Design review of the part built by this model. Coordinates are the model's own, in mm. A direction names the side the tool comes from. Coordinates: 2 decimals unless noted, no trailing zeros. Order: outer loops, then holes, each group sorted by start corner. A loop starts at its lowest first (then second) coordinate and runs counter-clockwise, first axis right, second up. Notation, with made-up numbers: M -5.5,8.5 L 31.5,8.5 A23 ccw 31.5,44.5 Z; hole C 83.25,-5 d3. An arc over 180 degrees is marked long. Use CSV: the item, a comma, the result in double quotes.
```python
from build123d import *

# Parameters (mm, degrees)
F1_DEPTH = 12.7
F2_W     = 101.6
F2_H     = 12.7
F3_DEPTH = 6.35
F4_R     = 5.08
F6_D     = 9.525
F8_D     = 6.35
F8_DEPTH = 5.08
F8_START = 0.3707141
F8_TIP   = 1.9077324654


with BuildPart() as f1:
    # F0 (on Front) → F1 (new body)
    with BuildSketch(Plane.XZ):
        Polygon((-101.6, 0), (0, 0), (0, 20.4238668084), (-18.1435327977, 20.4238668084), (-18.1435327977, 18.2426776737), (-15.169181861, 18.2426776737), (-13.1862824783, 16.259778291), (-5.8495542035, 16.259778291), (-5.8495542035, 13.2854273543), (-14.1777321696, 13.2854273543), (-20.5230116844, 5.9486986138), (-62.4783523381, 5.9486986138), (-96.535615623, 5.9486986138), (-99.9226495624, 13.2854273543), (-101.6, 13.2854273543), align=None)
    extrude(amount=F1_DEPTH)

    # F2 (on face) → F3 (join)
    with BuildSketch(Plane(origin=(0, 0, 0), x_dir=(1, 0, 0), z_dir=(0, 0, -1))):
        with Locations((-50.8, 6.35)):
            Rectangle(F2_W, F2_H)
    extrude(amount=F3_DEPTH)

    # F4
    f4_edges = [f1.edges().sort_by_distance(p)[0] for p in [
        (-50.8, -12.7, -6.35),
        (-50.8, 0, -6.35),
    ]]
    fillet(f4_edges, radius=F4_R)

    # F6 (through all)
    with Locations(Plane.YZ):
        with Locations((-6.35, 0)):
            Hole(F6_D / 2)

    # F8
    # its depths count from where the whole tool has entered the part; down to there all is cleared
    with Locations(Plane(origin=(0, 0, -6.35), x_dir=(1, 0, 0), z_dir=(0, 0, -1)).offset(-F8_START)):
        with Locations((-83.1515192986, 6.35)):
            Hole(F8_D / 2, depth=F8_DEPTH)
            with Locations((0, 0, -(F8_DEPTH + F8_TIP / 2))):  # 118° drill point
                Cone(0, F8_D / 2, F8_TIP, mode=Mode.SUBTRACT)


solid = f1.part
```
(1) For faces 1 (the face through (-18.144, -6, 19)), 2 (the face through (-58, -6, 5.949)), 3 (the face through (-10, -6, 16.26)), list the 3-axis set-ups (+Z, -Z, +X, -X, +Y, -Y) from which the entire face can be reached by the end or side of a thin tool; tool diameter is ignored.
The answers:
face 1,"+Z, -X, +Y, -Y"
face 2,"+Z, +Y, -Y"
face 3,"-X, +Y, -Y"
(2) Add section A-A on x = -9. Give the number of separate pieces and of enclosed holes in the cut face, and give its area (3 significant figures).
The answers:
separate pieces,"2"
enclosed holes,"1"
area,"220 mm2"
(3) Wall thickness on probe 1 along Z at (x, y) = (-92, -6); probe 2 along Z at (x, y) = (-71, -6.35); probe 3 along Z at (x, y) = (-9, -4): over which ranges is each line inside the solid? List them lowest first.
The answers:
probe 1,"z = -6.35 to -4.75, 4.75 to 5.95"
probe 2,"z = -6.35 to -4.76, 4.76 to 5.95"
probe 3,"z = -6.23 to -4.14, 4.14 to 13.29, 16.26 to 20.42"
(4) The part is to be moulded in two halves that separate along Z. For faces 4 (the face through (-98.205, -6.261, 9.566)), 5 (the face through (-50.089, -1.449, -4.822)), 6 (the face through (-40, 0, 5)), 7 (the face through (-17, -6, 18.243)), say which applies: pulls with the +Z half, pulls with the -Z half, needs draft (parallel to the pull), parting line crosses it, or undercut.
The answers:
face 4,"pulls with the +Z half"
face 5,"pulls with the -Z half"
face 6,"needs draft"
face 7,"undercut"
(5) Add section C-C on y = -6.35. State the section outline as (x, z) points, and give its area (3 significant figures).
The answers:
outline,"M -101.6,-6.35 L -86.33,-6.35 L -86.33,-4.76 L -101.6,-4.76 Z; M -101.6,4.76 L 0,4.76 L 0,20.42 L -18.14,20.42 L -18.14,18.24 L -15.17,18.24 L -13.19,16.26 L -5.85,16.26 L -5.85,13.29 L -14.18,13.29 L -20.52,5.95 L -96.54,5.95 L -99.92,13.29 L -101.6,13.29 Z; M -79.98,-6.35 L 0,-6.35 L 0,-4.76 L -79.98,-4.76 Z"
area,"509 mm2"
(6) Clearance check with flat-ended pins moving along their axes: P1, Ø2.5, axis at y = -7, z = 19, coming from the -X side; P2, Ø1, axis at x = -78, y = -10, coming from the +Z side; P3, Ø0.9, axis at y = -6.5, z = 14.5, coming from the -X side. State where each tip first meets the part, or that it passes through.
The answers:
P1,"stops at x = -18.14"
P2,"stops at z = 5.95"
P3,"stops at x = -5.85"
(7) Add section B-B on z = 0. State the section outline as (x, y) points.
The answers:
outline,"M -101.6,-12.7 L 0,-12.7 L 0,-11.11 L -101.6,-11.11 Z; M -101.6,-1.59 L 0,-1.59 L 0,0 L -101.6,0 Z"
